Check sheet for the modelled part. Datum: model origin and axes. Units: mm. Face numbers are marked on the shaded views. A direction names the side the tool comes from. Coordinates: 2 decimals unless noted, no trailing zeros. Loops run counter-clockwise (first coordinate to the right, second up) from the corner with the lowest first, then second, coordinate; pieces in that order, holes last. Notation, with made-up numbers: (72, 1) -> (130, 1) arc R21 cw to (130, 7) -> close; hole circle Ø3 at (-38.5, -32.5). An arc over 180 degrees is marked (long way). Use one line per item in the form item = value.
from build123d import *

# Parameters (mm, degrees)
SKETCH1_W           = 20
SKETCH1_H           = 11.25
BOSS_EXTRUDE1_DEPTH = 3
SKETCH1_3_W         = 20
SKETCH1_3_H         = 11.25
BOSS_EXTRUDE2_DEPTH = 15
SKETCH2_W           = 20
SKETCH2_H           = 11.25
CUT_EXTRUDE1_DEPTH  = 20
BOSS_EXTRUDE3_REACH = 58.127
SKETCH3_W           = 15
SKETCH3_H           = 5
SKETCH3_H_2         = 2.5
CUT_EXTRUDE2_REACH  = 58.844
SKETCH5_R           = 2
CUT_EXTRUDE3_DEPTH  = 57.844085005


with BuildPart() as part:
    # Sketch1 → Boss-Extrude1 (new body)
    with BuildSketch(Plane(origin=(0, 0, 0), x_dir=(1, 0, 0), z_dir=(0, 1, 0))):
        with BuildLine():
            Line((15, 11.25), (15, 22.5))
            Line((15, 22.5), (0, 22.5))
            Line((0, 22.5), (0, 11.25))
            Line((0, 11.25), (2, 11.25))
            ThreePointArc((2, 11.25), (4, 13.25), (6, 11.25))
            Line((6, 11.25), (8, 11.25))
            ThreePointArc((8, 11.25), (10, 13.25), (12, 11.25))
            Line((12, 11.25), (15, 11.25))
        make_face()
        with BuildLine():
            Line((0, 0), (15, 0))
            Line((15, 0), (15, 11.25))
            Line((15, 11.25), (12, 11.25))
            ThreePointArc((12, 11.25), (10, 9.25), (8, 11.25))
            Line((8, 11.25), (6, 11.25))
            ThreePointArc((6, 11.25), (4, 9.25), (2, 11.25))
            Line((2, 11.25), (0, 11.25))
            Line((0, 11.25), (0, 0))
        make_face()
        with Locations((25, 5.625)):
            Rectangle(SKETCH1_W, SKETCH1_H)
        with Locations((25, 16.875)):
            Rectangle(SKETCH1_W, SKETCH1_H)
        with BuildLine():
            Line((50, 11.25), (48, 11.25))
            ThreePointArc((48, 11.25), (46, 9.25), (44, 11.25))
            Line((44, 11.25), (42, 11.25))
            ThreePointArc((42, 11.25), (40, 9.25), (38, 11.25))
            Line((38, 11.25), (35, 11.25))
            Line((35, 11.25), (35, 0))
            Line((35, 0), (50, 0))
            Line((50, 0), (50, 11.25))
        make_face()
        with BuildLine():
            ThreePointArc((44, 11.25), (46, 13.25), (48, 11.25))
            Line((48, 11.25), (50, 11.25))
            Line((50, 11.25), (50, 22.5))
            Line((50, 22.5), (35, 22.5))
            Line((35, 22.5), (35, 11.25))
            Line((35, 11.25), (38, 11.25))
            ThreePointArc((38, 11.25), (40, 13.25), (42, 11.25))
            Line((42, 11.25), (44, 11.25))
        make_face()
    extrude(amount=BOSS_EXTRUDE1_DEPTH)

    # Sketch1<3> → Boss-Extrude2 (add)
    with BuildSketch(Plane(origin=(0, 0, 0), x_dir=(1, 0, 0), z_dir=(0, 1, 0))):
        with Locations((25, 5.625)):
            Rectangle(SKETCH1_3_W, SKETCH1_3_H)
        with Locations((25, 16.875)):
            Rectangle(SKETCH1_3_W, SKETCH1_3_H)
    extrude(amount=BOSS_EXTRUDE2_DEPTH)

    # Sketch2 → Cut-Extrude1 (cut)
    with BuildSketch(Plane.XY):
        with Locations((25, 7.625)):
            Rectangle(SKETCH2_W, SKETCH2_H)
    extrude(amount=-CUT_EXTRUDE1_DEPTH, mode=Mode.SUBTRACT)

    # Boss-Extrude3: up to this face of the body (flat: up to its plane)
    boss_extrude3_end = Plane(part.part.faces().sort_by_distance((25, 15, -11.25))[0])
    # Sketch3 → Boss-Extrude3 (add, up to the picked face)
    with BuildSketch(Plane(origin=(0, 3, 0), x_dir=(1, 0, 0), z_dir=(0, 1, 0)), mode=Mode.PRIVATE) as boss_extrude3_sk1:
        with Locations((42.5, 20)):
            Rectangle(SKETCH3_W, SKETCH3_H)
    boss_extrude3_tool1 = split(extrude(boss_extrude3_sk1.sketch, amount=BOSS_EXTRUDE3_REACH, mode=Mode.PRIVATE), bisect_by=boss_extrude3_end, keep=Keep.BOTH, mode=Mode.PRIVATE)
    # Sketch3 → Boss-Extrude3 (add, up to the picked face)
    with BuildSketch(Plane(origin=(0, 3, 0), x_dir=(1, 0, 0), z_dir=(0, 1, 0)), mode=Mode.PRIVATE) as boss_extrude3_sk2:
        with Locations((7.5, 20)):
            Rectangle(SKETCH3_W, SKETCH3_H)
    boss_extrude3_tool2 = split(extrude(boss_extrude3_sk2.sketch, amount=BOSS_EXTRUDE3_REACH, mode=Mode.PRIVATE), bisect_by=boss_extrude3_end, keep=Keep.BOTH, mode=Mode.PRIVATE)
    # Sketch3 → Boss-Extrude3 (add, up to the picked face)
    with BuildSketch(Plane(origin=(0, 3, 0), x_dir=(1, 0, 0), z_dir=(0, 1, 0)), mode=Mode.PRIVATE) as boss_extrude3_sk3:
        with Locations((7.5, 1.25)):
            Rectangle(SKETCH3_W, SKETCH3_H_2)
    boss_extrude3_tool3 = split(extrude(boss_extrude3_sk3.sketch, amount=BOSS_EXTRUDE3_REACH, mode=Mode.PRIVATE), bisect_by=boss_extrude3_end, keep=Keep.BOTH, mode=Mode.PRIVATE)
    # Sketch3 → Boss-Extrude3 (add, up to the picked face)
    with BuildSketch(Plane(origin=(0, 3, 0), x_dir=(1, 0, 0), z_dir=(0, 1, 0)), mode=Mode.PRIVATE) as boss_extrude3_sk4:
        with Locations((42.5, 1.25)):
            Rectangle(SKETCH3_W, SKETCH3_H_2)
    boss_extrude3_tool4 = split(extrude(boss_extrude3_sk4.sketch, amount=BOSS_EXTRUDE3_REACH, mode=Mode.PRIVATE), bisect_by=boss_extrude3_end, keep=Keep.BOTH, mode=Mode.PRIVATE)
    add(boss_extrude3_tool1.solids().sort_by(Axis((42.5, 3, -20), (0, 1, 0)))[0])
    add(boss_extrude3_tool2.solids().sort_by(Axis((7.5, 3, -20), (0, 1, 0)))[0])
    add(boss_extrude3_tool3.solids().sort_by(Axis((7.5, 3, -1.25), (0, 1, 0)))[0])
    add(boss_extrude3_tool4.solids().sort_by(Axis((42.5, 3, -1.25), (0, 1, 0)))[0])

    # Cut-Extrude2: up to this face of the body (flat: up to its plane)
    cut_extrude2_end = Plane(part.part.faces().sort_by_distance((25, 7.5, -22.5))[0])
    # Sketch4 → Cut-Extrude2 (cut, up to the picked face)
    with BuildSketch(Plane.XY, mode=Mode.PRIVATE) as cut_extrude2_sk1:
        Polygon((0, 4.75), (15, 15), (0, 15), align=None)
    cut_extrude2_tool1 = split(extrude(cut_extrude2_sk1.sketch, amount=-CUT_EXTRUDE2_REACH, mode=Mode.PRIVATE), bisect_by=cut_extrude2_end, keep=Keep.BOTH, mode=Mode.PRIVATE)
    # Sketch4 → Cut-Extrude2 (cut, up to the picked face)
    with BuildSketch(Plane.XY, mode=Mode.PRIVATE) as cut_extrude2_sk2:
        Polygon((50, 15), (35, 15), (50, 4.75), align=None)
    cut_extrude2_tool2 = split(extrude(cut_extrude2_sk2.sketch, amount=-CUT_EXTRUDE2_REACH, mode=Mode.PRIVATE), bisect_by=cut_extrude2_end, keep=Keep.BOTH, mode=Mode.PRIVATE)
    add(cut_extrude2_tool1.solids().sort_by(Axis((5, 11.583333, 0), (0, 0, -1)))[0], mode=Mode.SUBTRACT)
    add(cut_extrude2_tool2.solids().sort_by(Axis((45, 11.583333, 0), (0, 0, -1)))[0], mode=Mode.SUBTRACT)

    # Sketch5 → Cut-Extrude3 (cut, through all)
    with BuildSketch(Plane(origin=(0, 15, 0), x_dir=(1, 0, 0), z_dir=(0, 1, 0))):
        with Locations(Location((25, 11.25, 0), (0, 0, 270))):
            Circle(SKETCH5_R)
    extrude(amount=-CUT_EXTRUDE3_DEPTH, mode=Mode.SUBTRACT)


solid = part.part
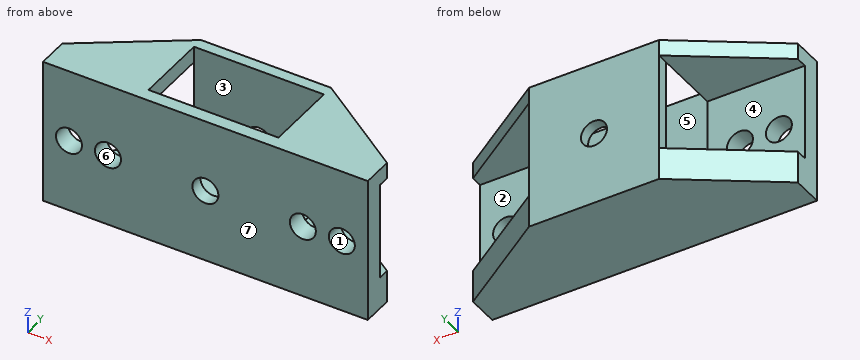
(1) Scan lines: line 1 along Y through (x, z) = (20.5, -2); line 2 along Z through (x, y) = (41, 5.5); line 3 along X through (y, z) = (14.45, -11.25). Record each from-to range of solid material in increasing order.
Established:
line_1 = 0 to 2, 13.25 to 15
line_2 = -22.5 to -17.5, -2.5 to 0
line_3 = 15 to 23, 27 to 35
(2) Section check C-C, the plane y = 7.75. Record the boundary of the cut face in (x, z), plus the area to 3 significant figures.
Established:
outline = (4.39, -22.5) -> (45.61, -22.5) -> (45.61, -17.5) -> (35, -17.5) -> (35, -20) -> (15, -20) -> (15, -17.5) -> (4.39, -17.5) -> close; (4.39, -2.5) -> (15, -2.5) -> (15, 0) -> (4.39, 0) -> close; (35, -2.5) -> (45.61, -2.5) -> (45.61, 0) -> (35, 0) -> close
area = 209 mm²
(3) Section check B-B, the plane x = 25. Record the boundary of the cut face in (y, z), plus the area to 3 significant figures.
Established:
outline = (0, -22.5) -> (15, -22.5) -> (15, -13.25) -> (13.25, -13.25) -> (13.25, -20) -> (2, -20) -> (2, -13.25) -> (0, -13.25) -> close; (0, -9.25) -> (2, -9.25) -> (2, 0) -> (0, 0) -> close; (13.25, -9.25) -> (15, -9.25) -> (15, 0) -> (13.25, 0) -> close
area = 97.5 mm²
(4) Section check A-A, the plane z = -14.25. Record the boundary of the cut face in (x, y), plus the area to 3 significant figures.
Established:
outline = (0, 0) -> (50, 0) -> (50, 3) -> (35, 3) -> (35, 2) -> (15, 2) -> (15, 3) -> (0, 3) -> close; (15, 13.25) -> (35, 13.25) -> (35, 15) -> (15, 15) -> close
area = 165 mm²
(5) Tool access check on the marked faces 1, 2 and 3. Record the directions out of +Z, -Z, +X, -X, +Y, -Y that give a thin tool (end or side, any length) a straight path to the whole face; none if there is none.
Established:
face_1 = +Y, -Y
face_2 = +X, -X, +Y
face_3 = +Z
(6) Go/stop test with flat-tipped pins: P1, Ø9, axis at x = 28.5, y = 7.5, coming from the +Z side; P2, Ø4.5, axis at x = 7, z = -10, coming from the +Y side; P3, Ø8, axis at y = 11.5, z = -11.5, coming from the +X side. Record where each tip stops, or that it passes through.
Established:
P1 = -20
P2 = 3
P3 = 35
(7) Section check D-D, the plane x = 4. Record the boundary of the cut face in (y, z).
Established:
outline = (0, -22.5) -> (7.48, -22.5) -> (7.48, -17.5) -> (3, -17.5) -> (3, -13.25) -> (0, -13.25) -> close; (0, -9.25) -> (3, -9.25) -> (3, -2.5) -> (7.48, -2.5) -> (7.48, 0) -> (0, 0) -> close
(8) Mould release check, pull along Y, two halves, no side actions. Record for the marked faces 4, 5, 6 and 7: +Y half, -Y half, draft (parallel to the pull), parting line (faces both ways), or undercut.
Established:
face_4 = +Y half
face_5 = undercut
face_6 = draft
face_7 = -Y half
